Check sheet for the modelled part. Datum: model origin and axes. Units: mm. Face numbers are marked on the shaded views. A direction names the side the tool comes from. Coordinates: 2 decimals unless noted, no trailing zeros. Write each loop counter-clockwise with the first axis right and the second up, starting at its lowest first coordinate (ties: lowest second). Pieces come first, ordered by that corner, then holes. Notation, with made-up numbers: (31.25, 72.25) -> (81.25, 72.25) arc R26 ccw to (81.25, 110.25) -> close; hole circle Ø4 at (48.5, 47). An arc over 180 degrees is marked (long way). One line per item, written item: value. Start each with the question number.
1) Gauge pin test, flat ends, axial feed: P1, Ø4.5, axis at x = 0, y = 0, coming from the +Z side; P2, Ø0.8, axis at x = 17.5, z = 1, coming from the +Y side; P3, Ø6, axis at x = 10, y = 4, coming from the -Z side; P4, Ø5, axis at y = 2, z = -7, coming from the +X side. Record the tip position at first contact, or that the pin passes through.
2) Sectioned sample at C-C on z = -11. Enter the section's corners in (x, y), plus the area to 3 significant figures.
3) Scan lines: line 1 along X through (y, z) = (0, -4.75); line 2 along Y through (x, z) = (21, 0.9); line 3 along Z through (x, y) = (8, -0.5). Record each from-to range of solid material in increasing order. Write a range as [from, to].
4) Sectioned sample at A-A on z = 0.5. Enter the section's corners in (x, y), plus the area to 3 significant figures.
5) Set-up check for the marked faces 1, 2, 3 and 4: record each of +Z, -Z, +X, -X, +Y, -Y from which the full face is reachable in a straight line by a thin tool's end or side.
6) Sectioned sample at B-B on y = 0. Enter the section's corners in (x, z), plus the area to 3 significant figures.
7) Draft check along X on the marked faces 5, 6 and 7. Enter one of: +X half, -X half, draft (parallel to the pull), parting line (faces both ways), or undercut.
```python
from build123d import *

# Parameters (mm, degrees)
SKETCH_1_W             = 50
SKETCH_1_H             = 8
EXTRUDE_484_DEPTH      = 2.75
SKETCH_6_R             = 4
EXTRUDE_752_DEPTH      = 12
HOLE_WIZARD_M3_D       = 2.5
HOLE_WIZARD_M2_D       = 1.6
EXTRUDE_3073_DEPTH     = 2.75
CUT_EXTRUDE_3452_DEPTH = 2.75
SKETCH_10_R            = 2.5
CUT_EXTRUDE_3895_DEPTH = 31.050948797
FILLET_4_RADIUS        = 4
FILLET_4_LENGTH        = 2.75
FILLET_5_RADIUS        = 4
FILLET_5_LENGTH        = 2.75
FILLET_6_R             = 2


with BuildPart() as part:
    # Эскиз1 → Extrude 484 (new body)
    with BuildSketch(Plane.XY):
        Rectangle(SKETCH_1_W, SKETCH_1_H)
    extrude(amount=EXTRUDE_484_DEPTH)

    # Эскиз6 → Extrude 752 (add)
    with BuildSketch(Plane(origin=(0, 0, 0), x_dir=(-1, 0, 0), z_dir=(0, 0, -1))):
        with Locations(Location((0, 0, 0), (0, 0, 270))):
            Circle(SKETCH_6_R)
    extrude(amount=EXTRUDE_752_DEPTH)

    # Крепление толкателей M3 (through all)
    with Locations(Plane.XY.offset(2.75)):
        with Locations((-21, 0), (21, 0)):
            Hole(HOLE_WIZARD_M3_D / 2)

    # Крепление вала M2 (through all)
    with Locations(Plane(origin=(0, 4, -5), x_dir=(1, 0, 0), z_dir=(0, 1, 0))):
        with Locations((0, 0)):
            Hole(HOLE_WIZARD_M2_D / 2)

    # Эскиз11 → Extrude 3073 (add)
    with BuildSketch(Plane.XY.offset(2.75)):
        with BuildLine():
            Line((-14, 0), (0, 0))
            Line((0, 0), (14, 0))
            ThreePointArc((14, 0), (0, 14), (-14, 0))
        make_face()
    extrude(amount=-EXTRUDE_3073_DEPTH)

    # Эскиз12 → Cut-Extrude 3452 (cut)
    with BuildSketch(Plane.XY.offset(2.75)):
        with BuildLine():
            Line((-5.986423051, 4), (5.986423051, 4))
            Line((5.986423051, 4), (11.640574572, 7.777983262))
            ThreePointArc((11.640574572, 7.777983262), (0, 14), (-11.640574572, 7.777983262))
            Line((-11.640574572, 7.777983262), (-5.986423051, 4))
        make_face()
    extrude(amount=-CUT_EXTRUDE_3452_DEPTH, mode=Mode.SUBTRACT)

    # Эскиз10 → Cut-Extrude 3895 (cut, through all)
    with BuildSketch(Plane.XY.offset(-12)):
        Circle(SKETCH_10_R)
    extrude(amount=CUT_EXTRUDE_3895_DEPTH, mode=Mode.SUBTRACT)

    # Скругление4: full round fillet: the end face becomes a half cylinder, R = half its width
    fillet_4_face = Plane((-25, 0, 1.375), x_dir=(0, 0, 1), z_dir=(-1, 0, 0))  # on the end face: x along it, z out of the body
    fillet_4_slab = fillet_4_face.offset(-FILLET_4_RADIUS / 2) * Box(FILLET_4_LENGTH, 2 * FILLET_4_RADIUS, FILLET_4_RADIUS, mode=Mode.PRIVATE)  # the body's end, R deep
    fillet_4_round = Plane((-21, 0, 1.375), x_dir=(-1, 0, 0), z_dir=(0, 0, 1)) * Cylinder(FILLET_4_RADIUS, FILLET_4_LENGTH, mode=Mode.PRIVATE)  # its axis R under the face
    add(fillet_4_slab - fillet_4_round, mode=Mode.SUBTRACT)

    # Скругление5: full round fillet: the end face becomes a half cylinder, R = half its width
    fillet_5_face = Plane((25, 0, 1.375), x_dir=(0, 0, 1), z_dir=(1, 0, 0))  # on the end face: x along it, z out of the body
    fillet_5_slab = fillet_5_face.offset(-FILLET_5_RADIUS / 2) * Box(FILLET_5_LENGTH, 2 * FILLET_5_RADIUS, FILLET_5_RADIUS, mode=Mode.PRIVATE)  # the body's end, R deep
    fillet_5_round = Plane((21, 0, 1.375), x_dir=(1, 0, 0), z_dir=(0, 0, 1)) * Cylinder(FILLET_5_RADIUS, FILLET_5_LENGTH, mode=Mode.PRIVATE)  # its axis R under the face
    add(fillet_5_slab - fillet_5_round, mode=Mode.SUBTRACT)

    # Скругление6
    fillet_6_edges = [part.edges().sort_by_distance(p)[0] for p in [
        (13.416407865, 4, 1.375),
        (-13.416407865, 4, 1.375),
        (5.986423051, 4, 1.375),
        (-5.986423051, 4, 1.375),
    ]]
    fillet(fillet_6_edges, radius=FILLET_6_R)


solid = part.part
```
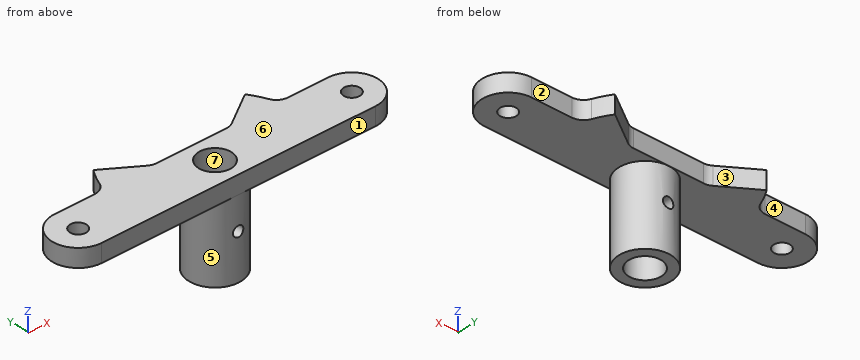
Answers:
1. P1: passes through
1. P2: stops at y = 4
1. P3: stops at z = 0
1. P4: stops at x = 4
2. outline: circle Ø8 at (0, 0); hole circle Ø5 at (0, 0)
2. area: 30.6 mm2
3. line 1: x = [-4, -2.5], [2.5, 4]
3. line 2: y = [-4, -1.25], [1.25, 4]
3. line 3: z = [0, 2.75]
4. outline: (-21, -4) -> (21, -4) arc R4 ccw to (21, 4) -> (14.83, 4) arc R2 cw to (12.98, 5.25) arc R14 ccw to (11.64, 7.78) -> (6.49, 4.34) arc R2 cw to (5.38, 4) -> (-5.38, 4) arc R2 cw to (-6.49, 4.34) -> (-11.64, 7.78) arc R14 ccw to (-12.98, 5.25) arc R2 cw to (-14.83, 4) -> (-21, 4) arc R4 ccw to start; hole circle Ø2.5 at (-21, 0); hole circle Ø5 at (0, 0); hole circle Ø2.5 at (21, 0)
4. area: 387 mm2
5. face 1: +Z, -Z, +X, -X, -Y
5. face 2: +Z, -Z, +X, +Y
5. face 3: +Z, -Z, +Y
5. face 4: +Z, -Z, -X, +Y
6. outline: (-25, 0) -> (-22.25, 0) -> (-22.25, 2.75) -> (-25, 2.75) -> close; (-19.75, 0) -> (-4, 0) -> (-4, -12) -> (-2.5, -12) -> (-2.5, 2.75) -> (-19.75, 2.75) -> close; (2.5, -12) -> (4, -12) -> (4, 0) -> (19.75, 0) -> (19.75, 2.75) -> (2.5, 2.75) -> close; (22.25, 0) -> (25, 0) -> (25, 2.75) -> (22.25, 2.75) -> close
6. area: 146 mm2
7. face 5: parting line
7. face 6: draft
7. face 7: undercut
